```python
from build123d import *

# Parameters (mm, degrees)
SKETCH2_W           = 76.2
SKETCH2_H           = 38.1
BOSS_EXTRUDE1_DEPTH = 12.7
BOSS_EXTRUDE2_START = 12.7
SKETCH2_3_W         = 76.2
SKETCH2_3_H         = 38.1
BOSS_EXTRUDE2_DEPTH = 12.7
CHAMFER1_SIZE       = 1.5875
SKETCH3_R           = 1.905
CUT_EXTRUDE1_DEPTH  = 58.15


with BuildPart() as part:
    # Sketch2 → Boss-Extrude1 (new body)
    # profile 1 of 2: a face of its own
    with BuildSketch(Plane.XY):
        with BuildLine():
            Line((-38.1, 25.4), (38.1, 25.4))
            ThreePointArc((38.1, 25.4), (42.590128061, 23.540128061), (44.45, 19.05))
            Line((44.45, 19.05), (44.45, -19.05))
            ThreePointArc((44.45, -19.05), (42.590128061, -23.540128061), (38.1, -25.4))
            Line((38.1, -25.4), (-38.1, -25.4))
            ThreePointArc((-38.1, -25.4), (-42.590128061, -23.540128061), (-44.45, -19.05))
            Line((-44.45, -19.05), (-44.45, 19.05))
            ThreePointArc((-44.45, 19.05), (-42.590128061, 23.540128061), (-38.1, 25.4))
        make_face()
        Rectangle(SKETCH2_W, SKETCH2_H, mode=Mode.SUBTRACT)
    # profile 2 of 2: a face of its own
    with BuildSketch(Plane.XY):
        Rectangle(SKETCH2_W, SKETCH2_H)
    extrude(amount=-BOSS_EXTRUDE1_DEPTH)

    # Sketch2_3 → Boss-Extrude2 (add)
    with BuildSketch(Plane.XY.offset(BOSS_EXTRUDE2_START)):
        with BuildLine():
            Line((-38.1, 25.4), (38.1, 25.4))
            ThreePointArc((38.1, 25.4), (42.590128061, 23.540128061), (44.45, 19.05))
            Line((44.45, 19.05), (44.45, -19.05))
            ThreePointArc((44.45, -19.05), (42.590128061, -23.540128061), (38.1, -25.4))
            Line((38.1, -25.4), (-38.1, -25.4))
            ThreePointArc((-38.1, -25.4), (-42.590128061, -23.540128061), (-44.45, -19.05))
            Line((-44.45, -19.05), (-44.45, 19.05))
            ThreePointArc((-44.45, 19.05), (-42.590128061, 23.540128061), (-38.1, 25.4))
        make_face()
        Rectangle(SKETCH2_3_W, SKETCH2_3_H, mode=Mode.SUBTRACT)
    extrude(amount=-BOSS_EXTRUDE2_DEPTH)

    # Chamfer1
    chamfer1_edges = [part.edges().sort_by_distance(p)[0] for p in [
        (-42.590128061, -23.540128061, 12.7),
        (0, -25.4, 12.7),
        (42.590128061, -23.540128061, 12.7),
        (44.45, 0, 12.7),
        (42.590128061, 23.540128061, 12.7),
        (0, 25.4, 12.7),
        (-42.590128061, 23.540128061, 12.7),
        (-44.45, 0, 12.7),
    ]]
    chamfer(chamfer1_edges, length=CHAMFER1_SIZE)

    # Sketch3 → Cut-Extrude1 (cut, through all)
    with BuildSketch(Plane(origin=(0, 0, -12.7), x_dir=(-1, 0, 0), z_dir=(0, 0, -1))):
        Circle(SKETCH3_R)
    extrude(amount=-CUT_EXTRUDE1_DEPTH, mode=Mode.SUBTRACT)


solid = part.part
```
Model file for the job. Use its own axes, mm. A direction names the side the tool comes from. Give positions to 0.01 mm unless a question says otherwise; leave off trailing zeros. Loops run counter-clockwise (first coordinate to the right, second up) from the corner with the lowest first, then second, coordinate; pieces in that order, holes last. Notation, with made-up numbers: (58, 3.5) - (86, 3.5) arc R34 ccw to (86, 39.5) - close; hole circle Ø5 at (23.25, 24). An arc over 180 degrees is marked (long way). One line per item, written item: value. Start each with the question number.
1. Slice it at D-D (y = -15.5). List the corners of the cut face in (x, z), plus the area to 3 significant figures.
2. Slice it at C-C (x = 28.5). List the corners of the cut face in (y, z).
3. Probe L1, parallel to X at y = -19, z = 4; L2, parallel to Y at x = 0, z = -6.75 (3 decimals); L3, parallel to Y at x = -36, z = 10.75. List the from-to ranges inside material, lowest first. Write a range as from..to.
4. Pull direction X, two halves, no side cores. Call faces 3 (the conical face through (-41.828, 22.697, 12.248)), 4 (the flat face through (1, 6, -12.7)), 5 (the cylindrical face through (0.41, -1.86, -6.44)): pulls with the +X half, pulls with the -X half, needs draft (parallel to the pull), parting line crosses it, or undercut.
5. Which spindle directions (+Z, -Z, +X, -X, +Y, -Y) get a long thin tool onto all of the face, cutting with end or side? Do faces 1 (the cylindrical face through (-42.54, -23.59, -0.63)), 2 (the flat face through (-1, 5, 0)). Say none if no direction does.
Solution:
1. outline: (-44.45, -12.7) - (44.45, -12.7) - (44.45, 11.11) - (42.86, 12.7) - (38.1, 12.7) - (38.1, 0) - (-38.1, 0) - (-38.1, 12.7) - (-42.86, 12.7) - (-44.45, 11.11) - close
1. area: 1,290 mm^2
2. outline: (-25.4, -12.7) - (25.4, -12.7) - (25.4, 11.11) - (23.81, 12.7) - (19.05, 12.7) - (19.05, 0) - (-19.05, 0) - (-19.05, 12.7) - (-23.81, 12.7) - (-25.4, 11.11) - close
3. L1: x = -44.45..-38.1, 38.1..44.45
3. L2: y = -25.4..-1.905, 1.905..25.4
3. L3: y = -25.4..-19.05, 19.05..25.4
4. face 3: pulls with the -X half
4. face 4: needs draft
4. face 5: undercut
5. face 1: +Z, -Z, -X, -Y
5. face 2: +Z
